from build123d import *

# Parameters (mm, degrees)
BOSS_EXTRUDE16_DEPTH = 3


with BuildPart() as part:
    # Sketch1 → Boss-Extrude16 (new body)
    with BuildSketch(Plane(origin=(0, 0, 0), x_dir=(1, 0, 0), z_dir=(0, 1, 0))):
        with BuildLine():
            Line((22.300293778, 0), (1.5, 0))
            Line((1.5, 0), (1.5, 5.3))
            ThreePointArc((1.5, 5.3), (0, 6.8), (-1.5, 5.3))
            Line((-1.5, 5.3), (-1.5, 0))
            Line((-1.5, 0), (-22.300293778, 0))
            ThreePointArc((-22.300293778, 0), (-23.468746199, 0.376818266), (-24.196904404, 1.365281059))
            Line((-24.196904404, 1.365281059), (-31.202449054, 22.298625838))
            ThreePointArc((-31.202449054, 22.298625838), (-31.335143696, 22.606562933), (-31.517418983, 22.888003588))
            Line((-31.517418983, 22.888003588), (-47.796410522, 43.921893905))
            ThreePointArc((-47.796410522, 43.921893905), (-48.161779402, 44.28546307), (-48.607932132, 44.543580677))
            Line((-48.607932132, 44.543580677), (-59.049183209, 48.9))
            ThreePointArc((-59.049183209, 48.9), (-64.537582367, 57.177202895), (-58.974890206, 65.404661131))
            ThreePointArc((-58.974890206, 65.404661131), (-57.197152686, 65.269831628), (-56.233330362, 63.769972896))
            Line((-56.233330362, 63.769972896), (-55.126688169, 53.675601541))
            ThreePointArc((-55.126688169, 53.675601541), (-54.747886441, 52.70603833), (-53.9331516, 52.058156621))
            Line((-53.9331516, 52.058156621), (-44.568394969, 48.00411216))
            ThreePointArc((-44.568394969, 48.00411216), (-44.155510387, 47.763109259), (-43.811617548, 47.431004165))
            Line((-43.811617548, 47.431004165), (-26.165884896, 25.744753421))
            ThreePointArc((-26.165884896, 25.744753421), (-25.988120723, 25.487567655), (-25.85260895, 25.205820999))
            Line((-25.85260895, 25.205820999), (-18.96208022, 7.444050869))
            ThreePointArc((-18.96208022, 7.444050869), (-17.421166495, 5.685274236), (-15.11, 5.33))
            Line((-15.11, 5.33), (-8.5424724, 6.639941055))
            ThreePointArc((-8.5424724, 6.639941055), (-7.828892036, 6.934141221), (-7.279856371, 7.476645151))
            Line((-7.279856371, 7.476645151), (-4.560453498, 11.47555039))
            ThreePointArc((-4.560453498, 11.47555039), (-3.880556824, 12), (-3.022136693, 12.020536776))
            Line((-3.022136693, 12.020536776), (0, 11.11))
            Line((0, 11.11), (3.022136693, 12.020536776))
            ThreePointArc((3.022136693, 12.020536776), (3.880556824, 12), (4.560453498, 11.47555039))
            Line((4.560453498, 11.47555039), (7.279856371, 7.476645151))
            ThreePointArc((7.279856371, 7.476645151), (7.828892036, 6.934141221), (8.5424724, 6.639941055))
            Line((8.5424724, 6.639941055), (15.11, 5.33))
            ThreePointArc((15.11, 5.33), (17.421166495, 5.685274236), (18.96208022, 7.444050869))
            Line((18.96208022, 7.444050869), (25.85260895, 25.205820999))
            ThreePointArc((25.85260895, 25.205820999), (25.988120723, 25.487567655), (26.165884896, 25.744753421))
            Line((26.165884896, 25.744753421), (43.811617548, 47.431004165))
            ThreePointArc((43.811617548, 47.431004165), (44.155510387, 47.763109259), (44.568394969, 48.00411216))
            Line((44.568394969, 48.00411216), (53.9331516, 52.058156621))
            ThreePointArc((53.9331516, 52.058156621), (54.747886441, 52.70603833), (55.126688169, 53.675601541))
            Line((55.126688169, 53.675601541), (56.233330362, 63.769972896))
            ThreePointArc((56.233330362, 63.769972896), (57.197152686, 65.269831628), (58.974890206, 65.404661131))
            ThreePointArc((58.974890206, 65.404661131), (64.537582367, 57.177202895), (59.049183209, 48.9))
            Line((59.049183209, 48.9), (48.607932132, 44.543580677))
            ThreePointArc((48.607932132, 44.543580677), (48.161779402, 44.28546307), (47.796410522, 43.921893905))
            Line((47.796410522, 43.921893905), (31.517418983, 22.888003588))
            ThreePointArc((31.517418983, 22.888003588), (31.335143696, 22.606562933), (31.202449054, 22.298625838))
            Line((31.202449054, 22.298625838), (24.196904404, 1.365281059))
            ThreePointArc((24.196904404, 1.365281059), (23.468746199, 0.376818266), (22.300293778, 0))
        make_face()
    extrude(amount=BOSS_EXTRUDE16_DEPTH)


solid = part.part
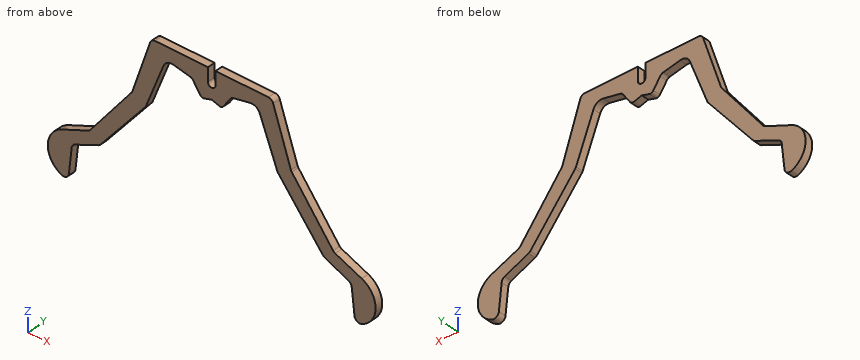
CAD build for the part. Positions are in the model's coordinates, mm. Coordinates: 2 decimals unless noted, no trailing zeros. Loops run counter-clockwise (first coordinate to the right, second up) from the corner with the lowest first, then second, coordinate; pieces in that order, holes last. Notation, with made-up numbers: (83, 45) - (109, 45) arc R19 ccw to (109, 81) - close; hole circle Ø10 at (10.25, -24). An arc over 180 degrees is marked (long way). Write item = value, one per line. Start each with the question number.
Q1. Cut at A-A, the plane z = -34.5. List the corners of the cut face in (x, y).
Q2. Drill centre lines: L1, parallel to X at y = 2.2, z = -9; L2, parallel to Z at x = 15, y = 2.95; L3, parallel to X at y = 0.5, z = -34. Where is each one in solid material? Low to high.
Q3. Flat gauge pins, fed straight in: pin 1 Ø1 at (y, z) = (1.5, -12.5) entering from -X; pin 2 Ø0.9 at (y, z) = (2, -3.5) entering from -X; pin 3 Ø12 at (x, z) = (6, -16.5) entering from +Y. Where does each tip first touch, or does it go through?
Q4. Cut at B-B, the plane z = -42.5. List the corners of the cut face in (x, y).
Computed:
q1.outline = (-40.5, 0) - (-33.29, 0) - (-33.29, 3) - (-40.5, 3) - close; (33.29, 0) - (40.5, 0) - (40.5, 3) - (33.29, 3) - close
q2.L1 = -26.75 to -19.57, -6.24 to 6.24, 19.57 to 26.75
q2.L2 = -5.35 to 0
q2.L3 = -40.12 to -32.88, 32.88 to 40.12
q3.pin_1 = -28.09
q3.pin_2 = -25.06
q3.pin_3 = 3
q4.outline = (-46.7, 0) - (-39.8, 0) - (-39.8, 3) - (-46.7, 3) - close; (39.8, 0) - (46.7, 0) - (46.7, 3) - (39.8, 3) - close
